from build123d import *

# Parameters (mm, degrees)
F0_W        = 190
F0_H        = 30
F1_DEPTH    = 4
F2_R        = 5
F3_DEPTH    = 20
F4_R        = 5.25
F5_DEPTH    = 2.3
F6_T1_DEPTH = 215.7168298797
F6_T3_DEPTH = 55.7168298797
F7_R        = 2.75
F8_DEPTH    = 75
F9_R        = 5


# Not quite as in the source:
# - a fillet or chamfer that OpenCascade refuses, or shapes differently, is made with other operations: its cross-section is extruded or revolved along the edge and cut away or added


with BuildPart() as f1:
    # F0 (on Top) → F1 (new body)
    with BuildSketch(Plane.XY):
        with Locations((1.5441179276, 0)):
            Rectangle(F0_W, F0_H)
    extrude(amount=-F1_DEPTH)

    # F2 (on Top) → F3 (join)
    with BuildSketch(Plane.XY):
        with Locations((-62.3, 0)):
            Circle(F2_R)
        with Locations((-31.15, 0)):
            Circle(F2_R)
        Circle(F2_R)
        with Locations((31.15, 0)):
            Circle(F2_R)
        with Locations((62.3, 0)):
            Circle(F2_R)
    extrude(amount=F3_DEPTH)

    # F4 (on face) → F5 (cut)
    with BuildSketch(Plane(origin=(0, 0, -4), x_dir=(1, 0, 0), z_dir=(0, 0, -1))):
        with Locations((-75, 0)):
            Circle(F4_R)
        Circle(F4_R)
        with Locations((75, 0)):
            Circle(F4_R)
    extrude(amount=-F5_DEPTH, mode=Mode.SUBTRACT)

    # F6: chamfer of 5 on 4 edges, made by hand

    # F6_s2 → F6_t1 (cut)
    with BuildSketch(Plane.YZ.offset(-106.3142970123)):
        Polygon((15, -5), (10, 0), (15, 0), align=None)
        Polygon((-10, 0), (-15, -5), (-15, 0), align=None)
    extrude(amount=F6_T1_DEPTH, mode=Mode.SUBTRACT)

    # F6_s4 → F6_t3 (cut)
    with BuildSketch(Plane.XZ.offset(-27.8584149398)):
        Polygon((96.5441179276, -5), (91.5441179276, 0), (96.5441179276, 0), align=None)
        Polygon((-93.4558820724, -5), (-88.4558820724, 0), (-93.4558820724, 0), align=None)
    extrude(amount=F6_T3_DEPTH, mode=Mode.SUBTRACT)

    # F7 (on Right) → F8 (cut, symmetric)
    with BuildSketch(Plane.YZ):
        with Locations((4.4393371791, 10)):
            Circle(F7_R)
    extrude(amount=F8_DEPTH, both=True, mode=Mode.SUBTRACT)

    # F9
    f9_edges = [f1.edges().sort_by_distance(p)[0] for p in [
        (-67.3, 0, 20),
        (-36.15, 0, 20),
        (-5, 0, 20),
        (26.15, 0, 20),
        (57.3, 0, 20),
    ]]
    fillet(f9_edges, radius=F9_R)


solid = f1.part
Source: CAD feature listing. Evaluate the final solid. Frame: model axes, mm. A direction names the side the tool comes from. Give positions to 0.01 mm unless a question says otherwise; leave off trailing zeros. Order: outer loops, then holes, each group sorted by start corner. A loop starts at its lowest first (then second) coordinate and runs counter-clockwise, first axis right, second up. Notation, with made-up numbers: (-23.75, -23) -> (18.25, -23) arc R19 cw to (18.25, -8) -> close; hole circle Ø8 at (1.5, -8). An arc over 180 degrees is marked (long way). Write item = value, one per line.
Item 1: Contact query for flat-ended pins moving along their axis: pin 1 (12 mm diameter, centred on x = 35, z = 9.5, fed in from -Y); pin 2 (5 mm diameter, centred on x = 73, y = 1, fed in from -Z); pin 3 (2 mm diameter, centred on y = 1, z = 4, fed in from +X). Output: stop coordinate, or through.
Check result:
pin_1 = -5
pin_2 = -1.7
pin_3 = 67.3
Item 2: Section query D-D (y = 12.25). Output: boundary loops of the cut face in (x, z).
Check result:
outline = (-92.46, -4) -> (95.54, -4) -> (93.79, -2.25) -> (-90.71, -2.25) -> close
Item 3: Section query A-A (z = 10). Output: boundary loops of the cut face in (x, y), then the cut area to 3 significant figures.
Check result:
outline = (-67.01, 1.69) arc R5 ccw (long way) to (-57.59, 1.69) -> close; (-35.86, 1.69) arc R5 ccw (long way) to (-26.44, 1.69) -> close; (-4.71, 1.69) arc R5 ccw (long way) to (4.71, 1.69) -> close; (26.44, 1.69) arc R5 ccw (long way) to (35.86, 1.69) -> close; (57.59, 1.69) arc R5 ccw (long way) to (67.01, 1.69) -> close
area = 279 mm²
Item 4: Section query C-C (z = 2). Output: boundary loops of the cut face in (x, y), then the cut area to 3 significant figures.
Check result:
outline = circle Ø10 at (-62.3, 0); circle Ø10 at (-31.15, 0); circle Ø10 at (0, 0); circle Ø10 at (31.15, 0); circle Ø10 at (62.3, 0)
area = 393 mm²
Item 5: Set-up query: faces 1 (the face through (-75, 0, -1.7)), 2 (the face through (93.572, 0.196, -2.028)), 3 (the face through (30.07, -4.88, 7.4)). Return all of +Z, -Z, +X, -X, +Y, -Y with unobstructed straight access to the full face (end or side cutting, diameter ignored); none if empty.
Check result:
face_1 = -Z
face_2 = +Z, +X, +Y, -Y
face_3 = +Z
Item 6: Section query B-B (x = 0). Output: boundary loops of the cut face in (y, z), then the cut area to 3 significant figures.
Check result:
outline = (-14, -4) -> (-5.25, -4) -> (-5.25, -1.7) -> (5.25, -1.7) -> (5.25, -4) -> (14, -4) -> (10, 0) -> (5, 0) -> (5, 7.31) arc R2.75 cw (long way) to (5, 12.69) -> (5, 15) arc R5 ccw to (-5, 15) -> (-5, 0) -> (-10, 0) -> close
area = 246 mm²
Item 7: Mould query, pull axis Y, two halves, no side actions, for faces 4 (the face through (0, 12, -2)), 5 (the face through (0, 6, -4)), 6 (the face through (-32.23, -4.88, 7.4)), 7 (the face through (75, 0, -1.7)). Classes: +Y half, -Y half, draft (parallel to the pull), parting line (faces both ways), or undercut.
Check result:
face_4 = +Y half
face_5 = draft
face_6 = parting line
face_7 = undercut
Item 8: Ray query, probe 1 along X at (y, z) = (-0.5, 13.5); probe 2 along X at (y, z) = (-4.5, 4.75); probe 3 along X at (y, z) = (0, -2.4). Return the intervals inside material, ascending.
Check result:
probe_1 = -67.27 to -57.33, -36.12 to -26.18, -4.97 to 4.97, 26.18 to 36.12, 57.33 to 67.27
probe_2 = -64.48 to -60.12, -33.33 to -28.97, -2.18 to 2.18, 28.97 to 33.33, 60.12 to 64.48
probe_3 = -90.86 to -80.25, -69.75 to -5.25, 5.25 to 69.75, 80.25 to 93.94
